```python
from build123d import *

# Parameters (mm, degrees)
F1_DEPTH = 8
F2_W     = 16
F2_H     = 76.1
F3_DEPTH = 5
F4_W     = 44
F4_H     = 76.1
F4_R     = 9.5
F5_DEPTH = 4


with BuildPart() as f1:
    # F0 (on Front) → F1 (new body)
    with BuildSketch(Plane.XZ):
        with BuildLine():
            ThreePointArc((-54.871013, -5.46831), (-59.871013, -0.46831), (-64.871013, -5.46831))
            ThreePointArc((-64.871013, -5.46831), (-59.871013, -10.46831), (-54.871013, -5.46831))
        make_face()
        Polygon((-37.871013, 32.58169), (-81.871013, 32.58169), (-81.871013, -5.46831), (-81.871013, -43.51831), (-37.871013, -43.51831), align=None)
        with BuildLine():
            ThreePointArc((-54.871013, -5.46831), (-59.871013, -10.46831), (-64.871013, -5.46831))
            ThreePointArc((-64.871013, -5.46831), (-59.871013, -0.46831), (-54.871013, -5.46831))
        make_face(mode=Mode.SUBTRACT)
    extrude(amount=F1_DEPTH)

    # F2 (on face) → F3 (join)
    with BuildSketch(Plane(origin=(-81.871013, 0, 0), x_dir=(0, -1, 0), z_dir=(-1, 0, 0))):
        with Locations((8, -5.46831)):
            Rectangle(F2_W, F2_H)
    extrude(amount=F3_DEPTH)

    # F4 (on face) → F5 (cut)
    with BuildSketch(Plane.XZ.offset(8)):
        with Locations((-59.871013, -5.46831)):
            Rectangle(F4_W, F4_H)
        with Locations((-59.871013, -5.46831)):
            Circle(F4_R, mode=Mode.SUBTRACT)
    extrude(amount=-F5_DEPTH, mode=Mode.SUBTRACT)


solid = f1.part
```
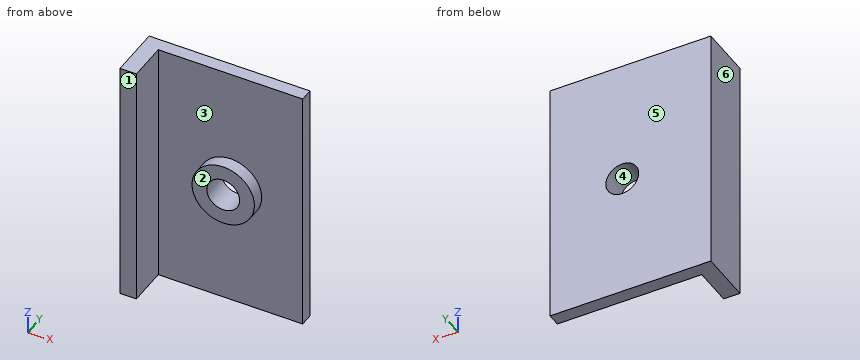
Read the model definition and answer for the solid it produces. Units are mm, in the model's axes. Face numbers are marked on the shaded views. A direction names the side the tool comes from. Round coordinates to 2 decimals unless told otherwise and drop trailing zeros. Write each loop counter-clockwise with the first axis right and the second up, starting at its lowest first coordinate (ties: lowest second). Pieces come first, ordered by that corner, then holes. Notation, with made-up numbers: (26, 57) - (81, 57) arc R16 cw to (81, 75) - close; hole circle Ø5 at (77, -29.5). An arc over 180 degrees is marked (long way). Use CSV: the item, a comma, the result in double quotes.
Q1. Each of these flat-tipped pins is pushed along its axis until it touches: pin 1 Ø9 at (x, z) = (-59.87, -5.47) entering from +Y; pin 2 Ø9.5 at (y, z) = (-7.5, -16.5) entering from +X; pin 3 Ø2 at (y, z) = (-12.5, 18.5) entering from +X; pin 4 Ø9.5 at (x, z) = (-58, -9.5) entering from -Y. Where does it stop, or does it pass through?
Values:
pin 1,"passes through"
pin 2,"stops at x = -37.87"
pin 3,"stops at x = -81.87"
pin 4,"stops at y = -8"
Q2. A tool of negligible diameter and unlimited length cuts with its end or side. For the marked faces 1, 2 and 3, from which of +Z, -Z, +X, -X, +Y, -Y can it reach the whole face along a straight path? Write none if from no direction.
Values:
face 1,"+Z, -Z, +X, -X, -Y"
face 2,"+Z, -Z, +X, -Y"
face 3,"-Y"
Q3. Determine the mould class of the marked faces 4, 5 and 6 for opening direction X: +X half, -X half, draft (parallel to the pull), parting line (faces both ways), or undercut.
Values:
face 4,"undercut"
face 5,"draft"
face 6,"-X half"
Q4. Find section A-A, the plane y = -5. Write down the section's boundary in (x, z).
Values:
outline,"(-86.87, -43.52) - (-81.87, -43.52) - (-81.87, 32.58) - (-86.87, 32.58) - close; circle Ø19 at (-59.87, -5.47); hole circle Ø10 at (-59.87, -5.47)"
Q5. Find section C-C, the plane z = -8. Write down the section's boundary in (x, y), then the cut area to 3 significant figures.
Values:
outline,"(-86.87, -16) - (-81.87, -16) - (-81.87, -4) - (-69.03, -4) - (-69.03, -8) - (-64.18, -8) - (-64.18, 0) - (-86.87, 0) - close; (-55.56, -8) - (-50.71, -8) - (-50.71, -4) - (-37.87, -4) - (-37.87, 0) - (-55.56, 0) - close"
area,"260 mm²"
Q6. Find section B-B, the plane x = -64. Write down the section's boundary in (y, z), then the cut area to 3 significant figures.
Values:
outline,"(-8, -14.02) - (-4, -14.02) - (-4, -43.52) - (0, -43.52) - (0, -8.29) - (-8, -8.29) - close; (-8, -2.65) - (0, -2.65) - (0, 32.58) - (-4, 32.58) - (-4, 3.09) - (-8, 3.09) - close"
area,"328 mm²"
Q7. Straight lines are drawn through the part: line 1 along X through (y, z) = (-5.75, -4.5); line 2 along X through (y, z) = (-4.75, -6); line 3 along Y through (x, z) = (-63.5, -33.5). For each, find the intervals that lie inside material, in ascending order.
Values:
line 1,"x = -86.87 to -81.87, -69.32 to -64.78, -54.97 to -50.42"
line 2,"x = -86.87 to -81.87, -69.36 to -64.84, -54.9 to -50.39"
line 3,"y = -4 to 0"
Q8. Find section D-D, the plane z = -32.5. Write down the section's boundary in (x, y), then the cut area to 3 significant figures.
Values:
outline,"(-86.87, -16) - (-81.87, -16) - (-81.87, -4) - (-37.87, -4) - (-37.87, 0) - (-86.87, 0) - close"
area,"256 mm²"
